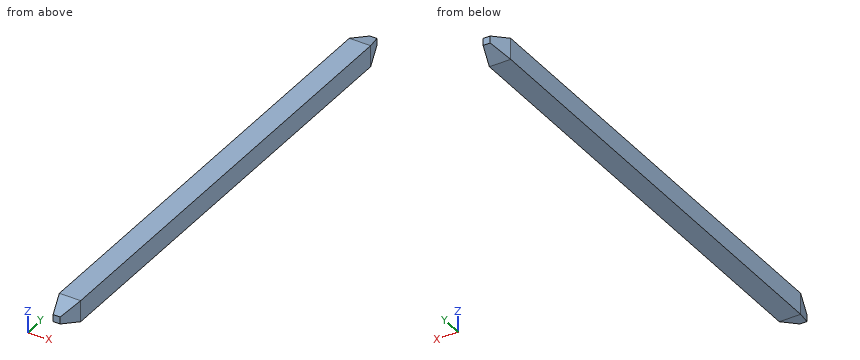
from build123d import *
from OCP.BRepFilletAPI import BRepFilletAPI_MakeChamfer

# Parameters (mm, degrees)
SKIZZE1_W                       = 0.6
SKIZZE1_H                       = 0.6
AUFSATZ_LINEAR_AUSTRAGEN1_DEPTH = 14.2
FASE1_SIZE                      = 0.6
FASE1_SIZE2                     = 0.2
FASE2_SIZE                      = 0.2
FASE2_SIZE2                     = 0.6


with BuildPart() as part:
    # Skizze1 → Aufsatz-Linear austragen1 (new body)
    with BuildSketch(Plane(origin=(0, 0, 0), x_dir=(1, 0, 0), z_dir=(0, 1, 0))):
        Rectangle(SKIZZE1_W, SKIZZE1_H)
    extrude(amount=AUFSATZ_LINEAR_AUSTRAGEN1_DEPTH)

    # Fase1: one chamfer whose edges measure the first distance from different faces: ONE call of the kernel's chamfer builder (chamfer() names one face for all edges)
    fase1_edges_1 = [part.edges().sort_by_distance(p)[0] for p in [
        (-0.3, 14.2, 0),
    ]]
    fase1_side_1 = [part.faces().sort_by_distance(p)[0] for p in [
        (-0.3, 7.1, 0),
    ]]
    fase1_edges_2 = [part.edges().sort_by_distance(p)[0] for p in [
        (0, 14.2, 0.3),
    ]]
    fase1_side_2 = [part.faces().sort_by_distance(p)[0] for p in [
        (0, 7.1, 0.3),
    ]]
    fase1_edges_3 = [part.edges().sort_by_distance(p)[0] for p in [
        (0.3, 14.2, 0),
    ]]
    fase1_side_3 = [part.faces().sort_by_distance(p)[0] for p in [
        (0.3, 7.1, 0),
    ]]
    fase1_edges_4 = [part.edges().sort_by_distance(p)[0] for p in [
        (0, 14.2, -0.3),
    ]]
    fase1_side_4 = [part.faces().sort_by_distance(p)[0] for p in [
        (0, 7.1, -0.3),
    ]]
    fase1 = BRepFilletAPI_MakeChamfer(part.part.solid().wrapped)
    for e in fase1_edges_1:
        fase1.Add(FASE1_SIZE, FASE1_SIZE2, e.wrapped, fase1_side_1[0].wrapped)  # the first distance lies on this face
    for e in fase1_edges_2:
        fase1.Add(FASE1_SIZE, FASE1_SIZE2, e.wrapped, fase1_side_2[0].wrapped)  # the first distance lies on this face
    for e in fase1_edges_3:
        fase1.Add(FASE1_SIZE, FASE1_SIZE2, e.wrapped, fase1_side_3[0].wrapped)  # the first distance lies on this face
    for e in fase1_edges_4:
        fase1.Add(FASE1_SIZE, FASE1_SIZE2, e.wrapped, fase1_side_4[0].wrapped)  # the first distance lies on this face
    add(Compound.cast(fase1.Shape()), mode=Mode.REPLACE)

    # Fase2
    fase2_edges = [part.edges().sort_by_distance(p)[0] for p in [
        (0, 0, 0.3),
        (-0.3, 0, 0),
        (0, 0, -0.3),
        (0.3, 0, 0),
    ]]
    fase2_side = [part.faces().sort_by_distance(p)[0] for p in [
        (0, 0, 0),
    ]]
    chamfer(fase2_edges, length=FASE2_SIZE, length2=FASE2_SIZE2, reference=fase2_side[0])


solid = part.part
Could you check a few things on this model? Use its own coordinates, in mm. Round coordinates to 2 decimals unless told otherwise and drop trailing zeros. Write each loop counter-clockwise with the first axis right and the second up, starting at its lowest first coordinate (ties: lowest second). Pieces come first, ordered by that corner, then holes. Notation, with made-up numbers: (46, -9) - (62, -9) arc R25 ccw to (62, 17) - close; hole circle Ø11 at (31.5, 13.5). An arc over 180 degrees is marked (long way). Put each result on its own line as item: value. Start each with the question number.
(1) I want a section at B-B, the plane z = 0. Please give me the cut outline in (x, y), plus the area to 3 significant figures.
(2) I need wall thicknesses on probe 1 along X at (y, z) = (13.75, 0.1). Which ranges of the line are inside material? Lowest first, please.
(3) I want a section at A-A, the plane x = 0.2. Please give me the cut outline in (y, z), plus the area to 3 significant figures.
Here are the results:
1. outline: (-0.3, 0.6) - (-0.1, 0) - (0.1, 0) - (0.3, 0.6) - (0.3, 13.6) - (0.1, 14.2) - (-0.1, 14.2) - (-0.3, 13.6) - close
1. area: 8.28 mm^2
2. probe 1: x = -0.25 to 0.25
3. outline: (0.3, -0.2) - (0.6, -0.3) - (13.6, -0.3) - (13.9, -0.2) - (13.9, 0.2) - (13.6, 0.3) - (0.6, 0.3) - (0.3, 0.2) - close
3. area: 8.10 mm^2
